from build123d import *

# Parameters (mm, degrees)
F1_DEPTH = 203.2


with BuildPart() as f1:
    # F0 (on Top) → F1 (new body)
    with BuildSketch(Plane.XY):
        Polygon((214.0153056353, 225.6372907119), (-192.3846943647, 225.6372907119), (-192.3846943647, -282.3627092881), (-141.5846943647, -282.3627092881), (163.2153056353, -282.3627092881), (214.0153056353, -282.3627092881), align=None)
        Polygon((163.2153056353, -282.3627092881), (-141.5846943647, -282.3627092881), (-141.5846943647, -470.7070589066), align=None)
        Polygon((-68.5457757791, -360.5891466141), (-80.6984541123, -360.5891466141), (-85.9086484415, -345.5981782754), (-108.2685105503, -345.5981782754), (-113.4787048795, -360.5891466141), (-125.7646362646, -360.5891466141), (-104.3508708244, -301.9178278628), (-89.866264083, -301.9178278628), align=None, mode=Mode.SUBTRACT)
        with BuildLine():
            add(Edge.make_bspline(
                [(-45.9926967451, -346.4243471972), (-41.5620327694, -351.7544692731), (-33.1937411102, -351.7544692731)],
                knots=[0, 0, 0, 1, 1, 1], degree=2))
            add(Edge.make_bspline(
                [(-33.1937411102, -351.7544692731), (-22.0671112766, -351.7544692731), (-17.7363870898, -340.6011888292)],
                knots=[0, 0, 0, 1, 1, 1], degree=2))
            Line((-17.7363870898, -340.6011888292), (-7.0361670223, -344.6387563017))
            add(Edge.make_bspline(
                [(-7.0361670223, -344.6387563017), (-10.4874210665, -353.1403010129), (-17.1767242718, -357.284470927)],
                knots=[0, 0, 0, 1, 1, 1], degree=2))
            add(Edge.make_bspline(
                [(-17.1767242718, -357.284470927), (-23.8660274772, -361.428640841), (-33.1937411102, -361.428640841)],
                knots=[0, 0, 0, 1, 1, 1], degree=2))
            add(Edge.make_bspline(
                [(-33.1937411102, -361.428640841), (-47.3452152219, -361.428640841), (-55.0672295794, -353.4068071167)],
                knots=[0, 0, 0, 1, 1, 1], degree=2))
            add(Edge.make_bspline(
                [(-55.0672295794, -353.4068071167), (-62.789243937, -345.3849733924), (-62.789243937, -330.980318482)],
                knots=[0, 0, 0, 1, 1, 1], degree=2))
            add(Edge.make_bspline(
                [(-62.789243937, -330.980318482), (-62.789243937, -316.5356876561), (-55.3403983358, -308.7870226882)],
                knots=[0, 0, 0, 1, 1, 1], degree=2))
            add(Edge.make_bspline(
                [(-55.3403983358, -308.7870226882), (-47.8915527347, -301.0383577202), (-33.7267533178, -301.0383577202)],
                knots=[0, 0, 0, 1, 1, 1], degree=2))
            add(Edge.make_bspline(
                [(-33.7267533178, -301.0383577202), (-23.3996417955, -301.0383577202), (-16.9035555155, -305.1825276343)],
                knots=[0, 0, 0, 1, 1, 1], degree=2))
            add(Edge.make_bspline(
                [(-16.9035555155, -305.1825276343), (-10.4074692354, -309.3266975484), (-7.7823841129, -317.3618565779)],
                knots=[0, 0, 0, 1, 1, 1], degree=2))
            Line((-7.7823841129, -317.3618565779), (-18.6158572324, -320.3200743301))
            add(Edge.make_bspline(
                [(-18.6158572324, -320.3200743301), (-19.9883636669, -315.9093983122), (-24.0059431817, -313.3043011476)],
                knots=[0, 0, 0, 1, 1, 1], degree=2))
            add(Edge.make_bspline(
                [(-24.0059431817, -313.3043011476), (-28.0235226965, -310.6992039829), (-33.4735725191, -310.6992039829)],
                knots=[0, 0, 0, 1, 1, 1], degree=2))
            add(Edge.make_bspline(
                [(-33.4735725191, -310.6992039829), (-41.8018882629, -310.6992039829), (-46.1126244918, -315.862759744)],
                knots=[0, 0, 0, 1, 1, 1], degree=2))
            add(Edge.make_bspline(
                [(-46.1126244918, -315.862759744), (-50.4233607207, -321.0263155052), (-50.4233607207, -330.980318482)],
                knots=[0, 0, 0, 1, 1, 1], degree=2))
            add(Edge.make_bspline(
                [(-50.4233607207, -330.980318482), (-50.4233607207, -341.0942251212), (-45.9926967451, -346.4243471972)],
                knots=[0, 0, 0, 1, 1, 1], degree=2))
        make_face(mode=Mode.SUBTRACT)
        Polygon((163.2153056353, -470.7070589066), (163.2153056353, -282.3627092881), (-141.5846943647, -470.7070589066), align=None)
        with BuildLine():
            add(Edge.make_bspline(
                [(85.7413243761, -400.5675143045), (93.8631018313, -408.0430141443), (93.8631018313, -421.9946154497)],
                knots=[0, 0, 0, 1, 1, 1], degree=2))
            add(Edge.make_bspline(
                [(93.8631018313, -421.9946154497), (93.8631018313, -431.0691526884), (90.3052436188, -437.8317483546)],
                knots=[0, 0, 0, 1, 1, 1], degree=2))
            add(Edge.make_bspline(
                [(90.3052436188, -437.8317483546), (86.7473854062, -444.5943440207), (80.2313080058, -448.1788528566)],
                knots=[0, 0, 0, 1, 1, 1], degree=2))
            add(Edge.make_bspline(
                [(80.2313080058, -448.1788528566), (73.7152306053, -451.7633616924), (65.2936336377, -451.7633616924)],
                knots=[0, 0, 0, 1, 1, 1], degree=2))
            Line((65.2936336377, -451.7633616924), (41.5612535758, -451.7633616924))
            Line((41.5612535758, -451.7633616924), (41.5612535758, -393.0920144647))
            Line((41.5612535758, -393.0920144647), (62.8018003578, -393.0920144647))
            add(Edge.make_bspline(
                [(62.8018003578, -393.0920144647), (77.6195469209, -393.0920144647), (85.7413243761, -400.5675143045)],
                knots=[0, 0, 0, 1, 1, 1], degree=2))
        make_face(mode=Mode.SUBTRACT)
        with BuildLine():
            add(Edge.make_bspline(
                [(117.7487229773, -437.5985554006), (122.1793891034, -442.9286800635), (130.5476848243, -442.9286800635)],
                knots=[0, 0, 0, 1, 1, 1], degree=2))
            add(Edge.make_bspline(
                [(130.5476848243, -442.9286800635), (141.6743200583, -442.9286800635), (146.0050463469, -431.7753942062)],
                knots=[0, 0, 0, 1, 1, 1], degree=2))
            Line((146.0050463469, -431.7753942062), (156.7052716079, -435.8129636385))
            add(Edge.make_bspline(
                [(156.7052716079, -435.8129636385), (153.2540158886, -444.3145124759), (146.5647094366, -448.4586844014)],
                knots=[0, 0, 0, 1, 1, 1], degree=2))
            add(Edge.make_bspline(
                [(146.5647094366, -448.4586844014), (139.8754029845, -452.6028563268), (130.5476848243, -452.6028563268)],
                knots=[0, 0, 0, 1, 1, 1], degree=2))
            add(Edge.make_bspline(
                [(130.5476848243, -452.6028563268), (116.3962038441, -452.6028563268), (108.6741857386, -444.5810187091)],
                knots=[0, 0, 0, 1, 1, 1], degree=2))
            add(Edge.make_bspline(
                [(108.6741857386, -444.5810187091), (100.9521676331, -436.5591810913), (100.9521676331, -422.1545191896)],
                knots=[0, 0, 0, 1, 1, 1], degree=2))
            add(Edge.make_bspline(
                [(100.9521676331, -422.1545191896), (100.9521676331, -407.7098813529), (108.4010168496, -399.9612126241)],
                knots=[0, 0, 0, 1, 1, 1], degree=2))
            add(Edge.make_bspline(
                [(108.4010168496, -399.9612126241), (115.8498660661, -392.2125438953), (130.014672358, -392.2125438953)],
                knots=[0, 0, 0, 1, 1, 1], degree=2))
            add(Edge.make_bspline(
                [(130.014672358, -392.2125438953), (140.3417888925, -392.2125438953), (146.8378783255, -396.3567158207)],
                knots=[0, 0, 0, 1, 1, 1], degree=2))
            add(Edge.make_bspline(
                [(146.8378783255, -396.3567158207), (153.3339677585, -400.5008877462), (155.9590541551, -408.5360506756)],
                knots=[0, 0, 0, 1, 1, 1], degree=2))
            Line((155.9590541551, -408.5360506756), (145.1255757776, -411.4942698636))
            add(Edge.make_bspline(
                [(145.1255757776, -411.4942698636), (143.7530686768, -407.083591705), (139.7354872121, -404.4784932759)],
                knots=[0, 0, 0, 1, 1, 1], degree=2))
            add(Edge.make_bspline(
                [(139.7354872121, -404.4784932759), (135.7179057474, -401.8733948469), (130.2678532795, -401.8733948469)],
                knots=[0, 0, 0, 1, 1, 1], degree=2))
            add(Edge.make_bspline(
                [(130.2678532795, -401.8733948469), (121.9395334936, -401.8733948469), (117.6287951724, -407.0369531142)],
                knots=[0, 0, 0, 1, 1, 1], degree=2))
            add(Edge.make_bspline(
                [(117.6287951724, -407.0369531142), (113.3180568512, -412.2005113814), (113.3180568512, -422.1545191896)],
                knots=[0, 0, 0, 1, 1, 1], degree=2))
            add(Edge.make_bspline(
                [(113.3180568512, -422.1545191896), (113.3180568512, -432.2684307376), (117.7487229773, -437.5985554006)],
                knots=[0, 0, 0, 1, 1, 1], degree=2))
        make_face(mode=Mode.SUBTRACT)
    extrude(amount=F1_DEPTH)


solid = f1.part
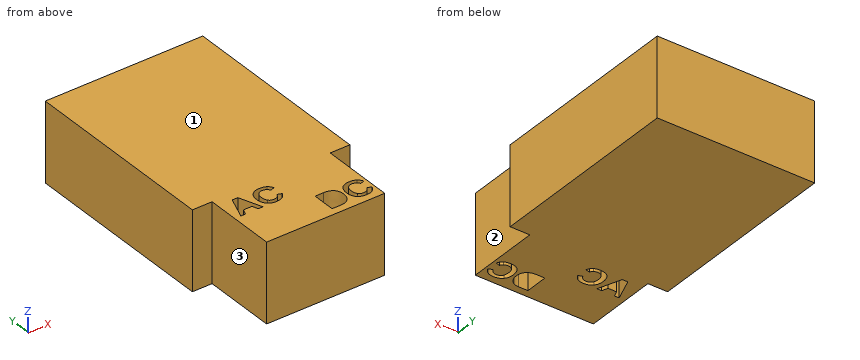
Verification items for the finished model (mm, model axes). Face numbers are marked on the shaded views. A direction names the side the tool comes from. Give positions to 0.01 mm unless a question says otherwise; leave off trailing zeros. Write each loop counter-clockwise with the first axis right and the second up, starting at its lowest first coordinate (ties: lowest second). Pieces come first, ordered by that corner, then holes.
(1) Gauge pin test, flat ends, axial feed: pin 1 (5 mm diameter, centred on y = -342.5, z = 44.5, fed in from -X); pin 2 (12 mm diameter, centred on x = -127, y = 115, fed in from -Z). Record the tip position at first contact, or that the pin passes through.
(2) Cross-section at B-B (z = 176). State how many separate pieces and enclosed holes the cut face has, plus the area to 3 significant figures.
(3) Cross-section at A-A (x = 187). Enter the section's corners in (y, z).
(4) Access from +Z, -Z, +X, -X, +Y, -Y to the whole of each face (thin tool, end or side, straight path). Record for the marked faces 1, 2 and 3.
(5) Material ranges on line 1 (Y direction, x = 134, z = 42); line 2 (Y direction, x = 52, z = 129); line 3 (Y direction, x = 138, z = 150.5), recorded low to high.
Worked out:
1. pin 1: stops at x = -141.58
1. pin 2: stops at z = 0
2. separate pieces: 1
2. enclosed holes: 4
2. area: 257,000 mm2
3. outline: (-282.36, 0) - (225.64, 0) - (225.64, 203.2) - (-282.36, 203.2) - close
4. face 1: +Z, +X, -X, +Y, -Y
4. face 2: +Z, -Z, +X, -Y
4. face 3: +Z, -Z, -X, -Y
5. line 1: y = -470.71 to -452.45, -442.63 to -402.21, -392.38 to 225.64
5. line 2: y = -470.71 to -451.76, -393.09 to 225.64
5. line 3: y = -470.71 to -451.85, -441.33 to -403.51, -392.94 to 225.64
